Read the model definition and answer for the solid it produces. Units are mm, in the model's axes. A direction names the side the tool comes from. Round coordinates to 2 decimals unless told otherwise and drop trailing zeros. Order: outer loops, then holes, each group sorted by start corner. A loop starts at its lowest first (then second) coordinate and runs counter-clockwise, first axis right, second up. Notation, with made-up numbers: (16, -28) - (42, -28) arc R16 cw to (42, 3) - close; hole circle Ø10 at (21, 19). An arc over 180 degrees is marked (long way). Answer as a JSON object with one key per item and string values. Group by question number.
Q1. The mould has two halves that part along X. Classify faces 3 (the flat face through (-17, -10, 39.6)), 4 (the cylindrical face through (18.504, 5.827, 35)), 5 (the cylindrical face through (17.264, 5.437, 11.154)): pulls with the +X half, pulls with the -X half, needs draft (parallel to the pull), parting line crosses it, or undercut.
Q2. A cutting plane is placed at B-B on z = 10. Determine the outline of the cut face in (x, y), and give its area (3 significant figures).
Q3. Consider line 1 (Z direction, x = -14.5, y = 17.5); line 2 (Y direction, x = 0, z = 6); line 3 (Y direction, x = -12, z = 47.5). Determine where each line is inside the solid, lowest interval first.
Q4. Given pin 1 Ø2 at (x, z) = (-17, 14) entering from +Y; pin 2 Ø2 at (x, z) = (14, 10) entering from -Y; pin 3 Ø8 at (y, z) = (-18.5, 15) entering from -X; pin 4 Ø4 at (x, y) = (11, -5) entering from -Z, each flat-ended and moving along its own axis, determine where each tip first touches the part or whether it passes through.
Q5. A tool of negligible diameter and unlimited length cuts with its end or side. For faces 1 (the flat face through (-15, -5, 61.5)), 2 (the cylindrical face through (-17.4, -13.3, 17.6)), from which of +Z, -Z, +X, -X, +Y, -Y can it reach the whole face along a straight path? Write none if from no direction.
Q6. A cutting plane is placed at A-A on z = 56. Determine the outline of the cut face in (x, y), and give its area (3 significant figures).
```python
from build123d import *


with BuildPart() as part:
    # Sketch (on XZ_Plane of Origin) → Revolution (revolve)
    with BuildSketch(Plane.XZ):
        Polygon((19.4, 61.5), (19.4, 31.5), (21.9, 22), (21.9, 0), (18.1, 0), (18.1, 22), (15.6, 31.5), (15.6, 61.5), align=None)
    revolve(axis=Axis((0, 0, 0), (0, 0, 1)))

    # Sketch001 (on XZ_Plane of Origin) → Revolution001 (revolve)
    with BuildSketch(Plane.XZ):
        Polygon((19.4, 61.5), (22.9, 61.5), (19.4, 58), align=None)
        Polygon((21.9, 3.6), (25.4, 0), (21.9, 0), align=None)
        Polygon((21.9, 13.3), (22.9, 13.3), (21.9, 12.3), align=None)
        Polygon((21.540092, 23.36765), (21.9, 22), (22.259908, 23.36765), align=None)
        Polygon((19.4, 49.3), (20.4, 49.3), (19.4, 48.3), align=None)
        Polygon((19.4, 39.6), (20.4, 39.6), (19.4, 38.6), align=None)
    revolve(axis=Axis((0, 0, 0), (0, 0, 1)))


solid = part.part
```
Result set:
{
 "1": {"face 3": "needs draft", "face 4": "parting line crosses it", "face 5": "undercut"},
 "2": {"outline": "circle Ø43.8 at (0, 0); hole circle Ø36.2 at (0, 0)", "area": "478 mm²"},
 "3": {"line 1": "z = 0 to 2.75, 13.13 to 13.3, 61.33 to 61.5", "line 2": "y = -21.9 to -18.1, 18.1 to 21.9", "line 3": "y = -15.24 to -9.97, 9.97 to 15.24"},
 "4": {"pin 1": "stops at y = 16.1", "pin 2": "stops at y = -17.62", "pin 3": "stops at x = -17.41", "pin 4": "passes through"},
 "5": {"face 1": "+Z, +X, -X, +Y, -Y", "face 2": "none"},
 "6": {"outline": "circle Ø38.8 at (0, 0); hole circle Ø31.2 at (0, 0)", "area": "418 mm²"}
}
